Autodesk Inventor part; units mm, degrees
ref_plane "Work Plane6" through (0, 5, 0) normal (0, 1, 0) x (1, 0, 0)
ref_plane "YZ Plane" through (0, 0, 0) normal (1, 0, 0) x (0, 1, 0)
ref_plane "XZ Plane" through (0, 0, 0) normal (0, 1, 0) x (-1, 0, 0)
sketch "Sketch1" plane through (0, 0, 0) normal (0, 1, 0) x (-1, 0, 0)
  line L0 (30, 30) -> (-30, 30)
  line L1 (-30, 30) -> (-30, -30)
  line L2 (-30, -30) -> (30, -30)
  line L3 (30, -30) -> (30, 30)
  line L4 (30, 30) -> (-30, -30) construction
  line L5 (-30, 30) -> (30, -30) construction
  point P0 (0, 0)
  dimension "d0" = 60
  dimension "d1" = 60
extrude "Extrusion1" add sketch "Sketch1" along normal blind 10
fillet "Fillet1" radius 7 4 edges at (30, 5, 30) (30, 5, -30) (-30, 5, 30) (-30, 5, -30)
sketch "Sketch2" plane through (0, 10, 0) normal (0, 1, 0) x (1, 0, 0)
  line L0 (-30, 30) -> (30, 30)
  line L1 (30, 30) -> (30, -30)
  line L2 (30, -30) -> (-30, -30)
  line L3 (-30, -30) -> (-30, 30)
  line L4 (-30, 30) -> (30, -30) construction
  line L5 (30, 30) -> (-30, -30) construction
  line L6 (25, -25) -> (25, 25)
  line L7 (25, 25) -> (-25, 25)
  line L8 (-25, 25) -> (-25, -25)
  line L9 (-25, -25) -> (25, -25)
  circle A0 centre (25, -25) radius 2.75
  circle A1 centre (-25, -25) radius 2.75
  circle A2 centre (25, 25) radius 2.75
  circle A3 centre (-25, 25) radius 2.75
  point P0 (0, 0)
  dimension "d5" = 5
  dimension "d6" = 5.5
  dimension "d7" = 5.5
  dimension "d8" = 5.5
  dimension "d9" = 5.5
extrude "Extrusion2" cut sketch "Sketch2" against normal blind 3 contours L9 A0 L6 | L6 A0 L9 | A2 L7 L6 | L6 L7 A2 | A1 L8 L9 | L9 L8 A1 | A3 L8 L7 | L7 L8 A3
sketch "Sketch7" plane through (0, 10, 0) normal (0, 1, 0) x (1, 0, 0)
  line L0 (-23, 30) -> (23, 30)
  line L1 (30, 23) -> (30, -23)
  line L2 (23, -30) -> (-23, -30)
  line L3 (-30, -23) -> (-30, 23)
  line L4 (-30, 30) -> (30, -30) construction
  line L5 (30, 30) -> (-30, -30) construction
  arc A0 (-23, 30) -> (-30, 23) centre (-23, 23) ccw
  arc A1 (-30, -23) -> (-23, -30) centre (-23, -23) ccw
  arc A2 (23, -30) -> (30, -23) centre (23, -23) ccw
  arc A3 (30, 23) -> (23, 30) centre (23, 23) ccw
  line L6 (23, 32) -> (-23, 32)
  arc A4 (-23, 32) -> (-32, 23) centre (-23, 23) ccw
  line L7 (-32, 23) -> (-32, -23)
  arc A5 (-32, -23) -> (-23, -32) centre (-23, -23) ccw
  line L8 (-23, -32) -> (23, -32)
  arc A6 (23, -32) -> (32, -23) centre (23, -23) ccw
  line L9 (32, -23) -> (32, 23)
  arc A7 (32, 23) -> (23, 32) centre (23, 23) ccw
  point P0 (0, 0)
  dimension "d47" = 7
  dimension "d48" = 2
extrude "Extrusion6" add sketch "Sketch7" against normal blind 10
sketch "Sketch23" plane through (0, 10, 0) normal (0, 1, 0) x (1, 0, 0)
  line L0 (-25, 25) -> (25, 25)
  line L1 (25, 25) -> (25, -25)
  line L2 (25, -25) -> (-25, -25)
  line L3 (-25, -25) -> (-25, 25)
  line L4 (-25, 25) -> (25, -25) construction
  line L5 (25, 25) -> (-25, -25) construction
  line L6 (21, -21) -> (21, 21)
  line L7 (21, 21) -> (-21, 21)
  line L8 (-21, 21) -> (-21, -21)
  line L9 (-21, -21) -> (21, -21)
  line L10 (-13.8, -15) -> (-13.8, 8.8)
  line L11 (-13.8, 8.8) -> (21, 8.8)
  line L12 (-11.8, 6.8) -> (-11.8, -15)
  line L13 (18, 8.8) -> (18, 6.8)
  line L14 (-13.8, -15) -> (18, -15)
  line L15 (7, 3.1073) -> (7, -15)
  line L16 (7, 3.1073) -> (7, 6.8)
  line L17 (5, -15) -> (5, 3.1073)
  line L18 (5, 3.1073) -> (5, 6.8)
  line L19 (5, 6.8) -> (-11.8, 6.8)
  line L20 (18, -15) -> (18, -18.6)
  line L21 (18, -18.6) -> (21, -18.6)
  line L22 (18, 6.8) -> (7, 6.8)
  point P0 (0, 0)
  point P1 (21, -15)
  dimension "d215" = 50
  dimension "d216" = 50
  dimension "d217" = 4
  dimension "d218" = 6
  dimension "d220" = 34.8
  dimension "d221" = 23.8
  dimension "d224" = 3
  dimension "d225" = 14
  dimension "d226" = 2
  dimension "d227" = 3
  dimension "d228" = 3.6
extrude "Extrusion21" cut sketch "Sketch23" against normal blind 2 contours L13 L22 L16 L15 L14 L17 L18 L19 L12 L10 L11
sketch "Sketch24" plane through (0, 10, 0) normal (0, 1, 0) x (1, 0, 0)
  line L0 (-11.8, 6.8) -> (5, 6.8)
  line L1 (5, 6.8) -> (5, -15)
  line L2 (5, -15) -> (-11.8, -15)
  line L3 (-11.8, -15) -> (-11.8, 6.8)
  point P0 (0, 0)
extrude "Extrusion22" cut sketch "Sketch24" against normal blind 8
sketch "Sketch25" plane through (0, 10, 0) normal (0, 1, 0) x (1, 0, 0)
  line L0 (7, 6.8) -> (18, 6.8)
  line L1 (18, 6.8) -> (18, 8.8)
  line L2 (18, 8.8) -> (21, 8.8)
  line L3 (7, 6.8) -> (7, -15)
  line L4 (21, 8.8) -> (21, -15)
  line L5 (7, -15) -> (18, -15)
  line L6 (18, -15) -> (18, -18.8)
  line L7 (18, -18.8) -> (21, -18.8)
  line L8 (21, -18.8) -> (21, -15)
  point P0 (0, 0)
  point P1 (21, -17.8036)
  dimension "d233" = 3
  dimension "d234" = 3
  dimension "d235" = 3.8
extrude "Extrusion23" cut sketch "Sketch25" against normal blind 8
sketch "Sketch26" plane through (0, 10, 0) normal (0, 1, 0) x (1, 0, 0)
  line L0 (23, 32) -> (-23, 32)
  line L1 (-32, 23) -> (-32, -23)
  line L2 (32, -23) -> (32, 23)
  line L3 (-13.8, 8.8) -> (21, 8.8)
  line L4 (-18, 28) -> (-18, 12.8)
  line L5 (-18, 12.8) -> (18, 12.8)
  line L6 (18, 12.8) -> (18, 28)
  line L7 (18, 28) -> (-18, 28)
  line L8 (-23, -32) -> (23, -32)
  line L9 (21, 8.8) -> (21, -18.8)
  line L10 (28, 18) -> (28, -18)
  line L11 (28, -18) -> (25, -18)
  line L12 (25, -18) -> (25, 8.8)
  line L13 (25, 8.8) -> (25, 12.8)
  line L14 (25, 12.8) -> (22, 12.8)
  line L15 (22, 12.8) -> (22, 18)
  line L16 (22, 18) -> (28, 18)
  line L17 (21, -18.8) -> (18, -18.8)
  line L18 (18, -15) -> (-13.8, -15)
  line L19 (18, -28) -> (-18, -28)
  line L20 (-18, -28) -> (-18, -19)
  line L21 (-18, -19) -> (13.8369, -19)
  line L22 (13.8369, -19) -> (13.8369, -22.8)
  line L23 (13.8369, -22.8) -> (18, -22.8)
  line L24 (18, -22.8) -> (18, -28)
  line L25 (-13.8, -15) -> (-13.8, 8.8)
  line L26 (-28, 18) -> (-22, 18)
  line L27 (-22, 18) -> (-22, 8.8)
  line L28 (-22, 8.8) -> (-17.8, 8.8)
  line L29 (-17.8, 8.8) -> (-17.8, -15)
  line L30 (-17.8, -15) -> (-22, -15)
  line L31 (-22, -15) -> (-22, -18)
  line L32 (-22, -18) -> (-28, -18)
  line L33 (-28, -18) -> (-28, 18)
  point P0 (0, 0)
  dimension "d238" = 4
  dimension "d239" = 4
  dimension "d240" = 14
  dimension "d241" = 14
  dimension "d242" = 4
  dimension "d243" = 4
  dimension "d244" = 14
  dimension "d245" = 4
  dimension "d246" = 14
  dimension "d247" = 4
  dimension "d248" = 4
  dimension "d249" = 4
  dimension "d250" = 4
  dimension "d251" = 14
  dimension "d252" = 14
  dimension "d253" = 4
  dimension "d254" = 4
  dimension "d255" = 4
  dimension "d256" = 14
  dimension "d257" = 4
  dimension "d258" = 14
  dimension "d259" = 4
  dimension "d260" = 4
extrude "Extrusion24" cut sketch "Sketch26" against normal through all
fillet "Fillet7" radius 0.5 13 edges at (-22, 5, -18) (-22, 5, -8.8) (-17.8, 5, -8.8) (-22, 5, 15) (-17.8, 5, 15) (-22, 5, 18) (22, 5, -12.8) (25, 5, -12.8) (28, 5, 18) (25, 5, 18) (13.8369, 5, 19) (13.8369, 5, 22.8) (18, 5, 22.8)
fillet "Fillet7" radius 1 5 edges at (22, 5, -18) (28, 5, -18) (-28, 5, -18) (-28, 5, 18) (18, 5, 28)
fillet "Fillet7" radius 2 6 edges at (-18, 5, -28) (18, 5, -28) (18, 5, -12.8) (-18, 5, -12.8) (-18, 5, 19) (-18, 5, 28)
ref_plane "Work Plane6" through (0, 5, 0) normal (0, 1, 0) x (1, 0, 0)
mirror "Mirror6" about plane through (0, 5, 0) normal (0, 1, 0) of "Extrusion2"
properties part number "16 pin holder"
Input: part model. Units: mm. Frame: model coordinates. A direction names the side the tool comes from. Give positions to 0.01 mm unless a question says otherwise; leave off trailing zeros. Write each loop counter-clockwise with the first axis right and the second up, starting at its lowest first coordinate (ties: lowest second). Pieces come first, ordered by that corner, then holes.
Q1. Section B-B, the plane z = 11.5. Output: boundary loops of the cut face in (x, y).
Q2. Section C-C, the plane z = -21. Output: boundary loops of the cut face in (x, y).
Q3. Section D-D, the plane x = -25. Output: boundary loops of the cut face in (y, z).
Q4. Section A-A, the plane x = -4. Output: boundary loops of the cut face in (y, z).
Q5. Set-up query: faces 1 (the face through (-17.43, 4.93, -27.4)), 2 (the face through (-25, 3, 25)), 3 (the face through (-4, 5, -6.8)). Return all of +Z, -Z, +X, -X, +Y, -Y with unobstructed straight access to the full face (end or side cutting, diameter ignored); none if empty.
Q6. Material intervals for probe 1 along Z at (x, y) = (-9, 2.75); probe 2 along X at (y, z) = (1.5, -10); probe 3 along X at (y, z) = (3.75, 8), sorted ascending.
Q7. First-contact query: P1, Ø3, axis at y = 3.5, z = 25.5, coming from the -X side; P2, Ø5, axis at x = -25, z = 25, coming from the +Y side; P3, Ø4.5, axis at x = -25, z = 25, coming from the -Y side. Flat tips, straight axial feed; report the tip coordinate or a pass-through.
Q8. Pull-direction query (X, two-part tool) for faces 4 (the face through (-27.747, 8.521, 24.879)), 5 (the face through (0, 5, 32)); classes: pulls with the +X half, pulls with the -X half, needs draft (parallel to the pull), parting line crosses it, or undercut.
Filled in:
1. outline: (-32, 0) - (-28, 0) - (-28, 10) - (-32, 10) - close; (-17.8, 0) - (25, 0) - (25, 10) - (21, 10) - (21, 2) - (7, 2) - (7, 8) - (5, 8) - (5, 2) - (-11.8, 2) - (-11.8, 8) - (-13.8, 8) - (-13.8, 10) - (-17.8, 10) - close; (28, 0) - (32, 0) - (32, 10) - (28, 10) - close
2. outline: (-32, 0) - (-18, 0) - (-18, 10) - (-32, 10) - close; (18, 0) - (32, 0) - (32, 10) - (18, 10) - close
3. outline: (0, -31.77) - (10, -31.77) - (10, -27.75) - (7, -27.75) - (7, -22.25) - (10, -22.25) - (10, -18) - (0, -18) - (0, -22.25) - (3, -22.25) - (3, -27.75) - (0, -27.75) - close; (0, 18) - (10, 18) - (10, 22.25) - (7, 22.25) - (7, 27.75) - (10, 27.75) - (10, 31.77) - (0, 31.77) - (0, 27.75) - (3, 27.75) - (3, 22.25) - (0, 22.25) - close
4. outline: (0, -32) - (10, -32) - (10, -28) - (0, -28) - close; (0, -12.8) - (10, -12.8) - (10, -8.8) - (8, -8.8) - (8, -6.8) - (2, -6.8) - (2, 15) - (10, 15) - (10, 19) - (0, 19) - close; (0, 28) - (10, 28) - (10, 32) - (0, 32) - close
5. face 1: +Y, -Y
5. face 2: -Y
5. face 3: +Y
6. probe 1: z = -32 to -28, -12.8 to -6.8, 15 to 19, 28 to 32
6. probe 2: x = -32 to -28, -22 to 25, 28 to 32
6. probe 3: x = -32 to -28, -17.8 to -11.8, 5 to 7, 21 to 25, 28 to 32
7. P1: stops at x = -31.94
7. P2: stops at y = 7
7. P3: stops at y = 3
8. face 4: undercut
8. face 5: needs draft
